from build123d import *

# Parameters (mm, degrees)
BOSS_EXTRUDE1_DEPTH     = 9.525
CUT_EXTRUDE1_DEPTH      = 13.494063522
CUT_EXTRUDE1_DEPTH_BACK = 13.494063522
SKETCH4_W               = 6.35
SKETCH4_H               = 2.9464
CUT_EXTRUDE3_DEPTH      = 13.494063522
CUT_EXTRUDE3_DEPTH_BACK = 13.494063522
SKETCH9_R               = 1.8034


with BuildPart() as part:
    # Sketch3 → Boss-Extrude1 (new, symmetric)
    with BuildSketch(Plane(origin=(0, 0, 0), x_dir=(0, 0, -1), z_dir=(1, 0, 0))):
        with BuildLine():
            Line((0, -1.4732), (-7.9502, -1.4732))
            Line((-7.9502, -1.4732), (-7.9502, -0.8382))
            Line((-7.9502, -0.8382), (0, -0.8382))
            ThreePointArc((0, -0.8382), (0.421388638, 0.724576328), (-0.728533124, -0.414510226))
            Line((-0.728533124, -0.414510226), (-1.280452157, -0.728533124))
            ThreePointArc((-1.280452157, -0.728533124), (0.740622455, 1.273497789), (0, -1.4732))
        make_face()
    extrude(amount=BOSS_EXTRUDE1_DEPTH, both=True)

    # Sketch4 → Cut-Extrude1 (cut, two sides: drawn at the far end of the back side and taken through both)
    with BuildSketch(Plane(origin=(0, 0, 0), x_dir=(1, 0, 0), z_dir=(0, 1, 0)).offset(-CUT_EXTRUDE1_DEPTH_BACK)):
        with Locations((-6.35, 0)):
            Rectangle(SKETCH4_W, SKETCH4_H)
        with Locations((6.35, 0)):
            Rectangle(SKETCH4_W, SKETCH4_H)
    extrude(amount=CUT_EXTRUDE1_DEPTH + CUT_EXTRUDE1_DEPTH_BACK, mode=Mode.SUBTRACT)

    # Cut-Extrude2 cone 1 section (through the dimple's axis) → Cut-Extrude2 (revolve, cut)
    with BuildSketch(Plane(origin=(5.5626, -0.8382, 4.7752), x_dir=(0, 0, 1), z_dir=(1, 0, 0))):
        Polygon((0, 0), (2.3114, 0), (0, 2.3114), align=None)
    revolve(axis=Axis((5.5626, -0.8382, 4.7752), (0, -1, 0)), mode=Mode.SUBTRACT)

    # Cut-Extrude2 cone 2 section (through the dimple's axis) → Cut-Extrude2 cone 2 (revolve, cut)
    with BuildSketch(Plane(origin=(-5.5626, -0.8382, 4.7752), x_dir=(0, 0, 1), z_dir=(1, 0, 0))):
        Polygon((0, 0), (2.3114, 0), (0, 2.3114), align=None)
    revolve(axis=Axis((-5.5626, -0.8382, 4.7752), (0, -1, 0)), mode=Mode.SUBTRACT)

    # Sketch9 → Cut-Extrude3 (cut, two sides: drawn at the far end of the back side and taken through both)
    with BuildSketch(Plane(origin=(0, 0, 0), x_dir=(1, 0, 0), z_dir=(0, 1, 0)).offset(-CUT_EXTRUDE3_DEPTH_BACK)):
        with Locations(Location((5.5626, -4.7752, 0), (0, 0, 270))):
            Circle(SKETCH9_R)
        with Locations(Location((-5.5626, -4.7752, 0), (0, 0, 270))):
            Circle(SKETCH9_R)
    extrude(amount=CUT_EXTRUDE3_DEPTH + CUT_EXTRUDE3_DEPTH_BACK, mode=Mode.SUBTRACT)


solid = part.part
Work out the finished part from the listing and answer in its coordinate system (mm). A direction names the side the tool comes from. Give positions to 0.01 mm unless a question says otherwise; leave off trailing zeros. Order: outer loops, then holes, each group sorted by start corner. A loop starts at its lowest first (then second) coordinate and runs counter-clockwise, first axis right, second up. Notation, with made-up numbers: M -18.5,-27.75 L -6.5,-27.75 A13 cw -6.5,-13.75 Z; hole C 12,53.25 d3. An arc over 180 degrees is marked long. Return JSON: item names as keys, results as strings.
Q1. Find section B-B, the plane x = -0.25. Write down the section's boundary in (y, z), and give its area (3 significant figures).
Answer below:
{"outline": "M -1.47,0 A1.47 ccw long -0.73,1.28 L -0.41,0.73 A0.84 cw long -0.84,0 L -0.84,7.95 L -1.47,7.95 Z", "area": "8.89 mm^2"}
Q2. Which of the six approach directions +Z, -Z, +X, -X, +Y, -Y give full straight-line access (tool end or side, diameter ignored) to faces 1 (the face through (-3.175, -1, 0)), 2 (the face through (3.175, -1, 0)), 3 (the face through (0, -0.838, 4))?
Answer below:
{"face 1": "-Z, -X, +Y, -Y", "face 2": "-Z, +X, +Y, -Y", "face 3": "+Z, +X, -X"}
Q3. This flat-tipped pin is pushed along its axis until it touches: pin 1 (2.5 mm diameter, centred on x = -0.5, z = 3, fed in from +Y). Where does it stop, or does it pass through?
Answer below:
{"pin 1": "stops at y = -0.84"}
Q4. Find section D-D, the plane y = 1.2. Write down the section's boundary in (x, z) (3 decimals).
Answer below:
{"outline": "M -3.175,-0.855 L 3.175,-0.855 L 3.175,0.855 L -3.175,0.855 Z"}
Q5. Find section C-C, the plane z = 2. Write down the section's boundary in (x, y) (3 decimals).
Answer below:
{"outline": "M -9.525,-1.473 L 9.525,-1.473 L 9.525,-0.838 L -9.525,-0.838 Z"}
Q6. Find the intervals of material crossed by line 1 along Y through (x, z) = (-0.5, 0); line 2 along X through (y, z) = (-1.3, 6) (3 decimals), in increasing order. Write a range as [from, to].
Answer below:
{"line 1": "y = [-1.47, -0.84], [0.84, 1.47]", "line 2": "x = [-9.525, -6.949], [-4.177, 4.177], [6.949, 9.525]"}
Q7. Find section A-A, the plane y = 0. Write down the section's boundary in (x, z) (3 decimals).
Answer below:
{"outline": "M -3.175,-1.473 L 3.175,-1.473 L 3.175,-0.838 L -3.175,-0.838 Z; M -3.175,0.838 L 3.175,0.838 L 3.175,1.473 L -3.175,1.473 Z"}
